Build history of the part. All positions in model axes, mm. A direction names the side the tool comes from. Round coordinates to 2 decimals unless told otherwise and drop trailing zeros. Order: outer loops, then holes, each group sorted by start corner. A loop starts at its lowest first (then second) coordinate and runs counter-clockwise, first axis right, second up. Notation, with made-up numbers: M 26.5,14 L 77.5,14 A23 cw 77.5,44 Z; hole C 65,-31 d9. An arc over 180 degrees is marked long. One line per item, written item: value. Start each with the question number.
Item 1: Tool access for faces 1 (the flat face through (0, 8, -10.16)), 2 (the cylindrical face through (-1.323, -6.619, 10.074)), 3 (the flat face through (10, 0, -10)): list every direction of +Z, -Z, +X, -X, +Y, -Y with a clear straight run to the whole face (end or side of a thin tool).
Item 2: Probe L1, parallel to Z at x = -2.54, y = 1.65 (3 decimals); L2, parallel to Z at x = 5.08, y = 1.7 (3 decimals). List the from-to ranges inside material, lowest first.
Item 3: Band-saw the part on A-A, the plane y = 11. Write the cut outline in (x, z), then the cut area to 3 significant figures.
Item 4: Two-plate mould, pull along Z, no slides. Class faces 4 (the flat face through (-10, 0, 10)), 5 (the flat face through (0, -3.175, 0)), 6 (the flat face through (0, 6, -12.7)): +Z half, -Z half, draft (parallel to the pull), parting line (faces both ways), or undercut.
Item 5: Band-saw the part on B-B, the plane z = 2.54. Give the number of separate pieces and of enclosed holes in the cut face, then the cut area to 3 significant figures.
Item 6: Pin check, flat tips, straight feed: pin 1 (1 mm diameter, centred on x = 5, y = -6, fed in from -Z); pin 2 (1 mm diameter, centred on x = 0, z = -5.08, fed in from +Y); pin 3 (12 mm diameter, centred on x = 0, z = 0, fed in from +Y); pin 4 (5 mm diameter, centred on y = -6, z = -7.5, fed in from +X). Stop position of each tip, or through.
```python
from build123d import *

# Parameters (mm, degrees)
F0_R     = 12.7
F0_R_2   = 10.16
F1_DEPTH = 12.7
F0_R_3   = 0.635
F2_DEPTH = 3.175
F4_DEPTH = 12.7
F3_R     = 0.635
F5_DEPTH = 2.54


# Not quite as in the source:
# - a fillet or chamfer that OpenCascade refuses, or shapes differently, is made with other operations: its cross-section is extruded or revolved along the edge and cut away or added


with BuildPart() as f1:
    # F0 (on Front) → F1 (new body)
    with BuildSketch(Plane.XZ):
        Circle(F0_R)
        Circle(F0_R_2, mode=Mode.SUBTRACT)
    extrude(amount=F1_DEPTH)

    # F0 (on Front) → F2 (join)
    with BuildSketch(Plane.XZ):
        Circle(F0_R_2)
        with Locations((0, -5.08)):
            Circle(F0_R_3, mode=Mode.SUBTRACT)
        with Locations((-5.08, 0)):
            Circle(F0_R_3, mode=Mode.SUBTRACT)
        with Locations((-2.54, -2.54)):
            Circle(F0_R_3, mode=Mode.SUBTRACT)
        with Locations((2.54, -2.54)):
            Circle(F0_R_3, mode=Mode.SUBTRACT)
        with Locations((5.08, 0)):
            Circle(F0_R_3, mode=Mode.SUBTRACT)
        with Locations((-2.54, 2.54)):
            Circle(F0_R_3, mode=Mode.SUBTRACT)
        with Locations((0, 5.08)):
            Circle(F0_R_3, mode=Mode.SUBTRACT)
        with Locations((2.54, 2.54)):
            Circle(F0_R_3, mode=Mode.SUBTRACT)
    extrude(amount=F2_DEPTH)

    # F3 (on face) → F4 (join)
    with BuildSketch(Plane(origin=(0, 0, 0), x_dir=(-1, 0, 0), z_dir=(0, 1, 0))):
        with BuildLine():
            ThreePointArc((-7.62, 10.16), (-4.0160926196, 12.0482778882), (1.86e-08, 12.7))
            Line((1.86e-08, 12.7), (-12.7, 12.7))
            Line((-12.7, 12.7), (-12.7, 10.16))
            Line((-12.7, 10.16), (-7.62, 10.16))
        make_face()
        with BuildLine():
            ThreePointArc((7.62, 10.16), (4.0160926372, 12.0482778823), (1.86e-08, 12.7))
            ThreePointArc((1.86e-08, 12.7), (-4.0160926196, 12.0482778882), (-7.62, 10.16))
            Line((-7.62, 10.16), (7.62, 10.16))
        make_face()
        with BuildLine():
            Line((12.7, 10.16), (12.7, 12.7))
            Line((12.7, 12.7), (1.86e-08, 12.7))
            ThreePointArc((1.86e-08, 12.7), (4.0160926372, 12.0482778823), (7.62, 10.16))
            Line((7.62, 10.16), (12.7, 10.16))
        make_face()
        with BuildLine():
            Line((12.7, -12.7), (12.7, -10.16))
            Line((12.7, -10.16), (7.62, -10.16))
            ThreePointArc((7.62, -10.16), (4.0160926284, -12.0482778852), (0, -12.7))
            Line((0, -12.7), (12.7, -12.7))
        make_face()
        with BuildLine():
            ThreePointArc((0, -12.7), (4.0160926284, -12.0482778852), (7.62, -10.16))
            Line((7.62, -10.16), (-7.62, -10.16))
            ThreePointArc((-7.62, -10.16), (-4.0160926284, -12.0482778852), (0, -12.7))
        make_face()
        with BuildLine():
            Line((-7.62, -10.16), (-12.7, -10.16))
            Line((-12.7, -10.16), (-12.7, -12.7))
            Line((-12.7, -12.7), (0, -12.7))
            ThreePointArc((0, -12.7), (-4.0160926284, -12.0482778852), (-7.62, -10.16))
        make_face()
    extrude(amount=F4_DEPTH)

    # F3 (on face) → F5 (join)
    with BuildSketch(Plane(origin=(0, 0, 0), x_dir=(-1, 0, 0), z_dir=(0, 1, 0))):
        with BuildLine():
            Line((12.7, 0), (12.7, 10.16))
            Line((12.7, 10.16), (7.62, 10.16))
            ThreePointArc((7.62, 10.16), (11.3592253257, 5.6796126628), (12.7, 0))
        make_face()
        with BuildLine():
            ThreePointArc((12.7, 0), (11.3592253257, 5.6796126628), (7.62, 10.16))
            Line((7.62, 10.16), (-7.62, 10.16))
            ThreePointArc((-7.62, 10.16), (-11.3592253257, 5.6796126628), (-12.7, 0))
            ThreePointArc((-12.7, 0), (-11.3592253257, -5.6796126628), (-7.62, -10.16))
            Line((-7.62, -10.16), (7.62, -10.16))
            ThreePointArc((7.62, -10.16), (11.3592253257, -5.6796126628), (12.7, 0))
        make_face()
        with Locations((0, -5.08)):
            Circle(F3_R, mode=Mode.SUBTRACT)
        with Locations((-5.08, 0)):
            Circle(F3_R, mode=Mode.SUBTRACT)
        with Locations((-2.54, -2.54)):
            Circle(F3_R, mode=Mode.SUBTRACT)
        with Locations((2.54, -2.54)):
            Circle(F3_R, mode=Mode.SUBTRACT)
        with Locations((5.08, 0)):
            Circle(F3_R, mode=Mode.SUBTRACT)
        with Locations((-2.54, 2.54)):
            Circle(F3_R, mode=Mode.SUBTRACT)
        with Locations((0, 5.08)):
            Circle(F3_R, mode=Mode.SUBTRACT)
        with Locations((2.54, 2.54)):
            Circle(F3_R, mode=Mode.SUBTRACT)
        with BuildLine():
            ThreePointArc((-12.7, 0), (-11.3592253257, 5.6796126628), (-7.62, 10.16))
            Line((-7.62, 10.16), (-12.7, 10.16))
            Line((-12.7, 10.16), (-12.7, 0))
        make_face()
        with BuildLine():
            Line((12.7, -10.16), (12.7, 0))
            ThreePointArc((12.7, 0), (11.3592253257, -5.6796126628), (7.62, -10.16))
            Line((7.62, -10.16), (12.7, -10.16))
        make_face()
        with BuildLine():
            ThreePointArc((-7.62, -10.16), (-11.3592253257, -5.6796126628), (-12.7, 0))
            Line((-12.7, 0), (-12.7, -10.16))
            Line((-12.7, -10.16), (-7.62, -10.16))
        make_face()
    extrude(amount=F5_DEPTH)

    # F6: chamfer of 5.08 on 1 edges, made by hand

    # F6_s1 → F6_t2 (revolve, cut)
    with BuildSketch(Plane.XY):
        Polygon((12.7, -7.62), (7.62, -12.7), (12.7, -12.7), align=None)
    revolve(axis=Axis((0, -12.7, 0), (0, -1, 0)), mode=Mode.SUBTRACT)


solid = f1.part
```
Output:
1. face 1: +X, -X, +Y
1. face 2: -Y
1. face 3: -Z, +X, -Y
2. L1: z = -12.7 to -3.175, -1.905 to 1.905, 3.175 to 12.7
2. L2: z = -12.7 to -0.635, 0.635 to 12.7
3. outline: M -12.7,-12.7 L 12.7,-12.7 L 12.7,-10.16 L -12.7,-10.16 Z; M -12.7,10.16 L 12.7,10.16 L 12.7,12.7 L -12.7,12.7 Z
3. area: 129 mm²
4. face 4: draft
4. face 5: undercut
4. face 6: -Z half
5. separate pieces: 3
5. enclosed holes: 0
5. area: 159 mm²
6. pin 1: stops at z = -11.88
6. pin 2: passes through
6. pin 3: stops at y = 2.54
6. pin 4: stops at x = 11.67
